Part print with two shaded views. Sizes in mm from the minimum x, y, z corner. Round coordinates to 2 decimals unless told otherwise and drop trailing zeros. Write each loop counter-clockwise with the first axis right and the second up, starting at its lowest first coordinate (ties: lowest second). Pieces come first, ordered by that corner, then holes. Notation, with made-up numbers: (42, 42) -> (52, 42) arc R18 cw to (52, 75) -> close; hole circle Ø3 at (70.25, -36.75). An arc over 180 degrees is marked (long way). Return JSON: item names as keys, results as strings. Group by question number.
(1) Saw through at A-A (x = 19.3). List the corners of the cut face in (y, z).
(2) Drill centre lines: L1, parallel to Y at x = 19.3, z = 2.6; L2, parallel to Y at x = 19.3, z = 0.7; L3, parallel to Y at x = 4, z = 2 (1 decimal). Where is each one in solid material? Low to high. Write a range as from..to.
(3) Mould opens along Y. For the marked faces 1, 2 and 3 say: +Y half, -Y half, draft (parallel to the pull), parting line (faces both ways), or undercut.
(4) Saw through at B-B (y = 19.3). List the corners of the cut face in (x, z).
(5) Saw through at C-C (z = 1.1). List the corners of the cut face in (x, y).
(6) Saw through at D-D (y = 28). List the corners of the cut face in (x, z) (1 decimal).
(7) Drop flat-ended pins along their axis: pin 1 Ø1 at (x, z) = (7, 0.5) entering from -Y; pin 2 Ø1 at (x, z) = (27.5, 2.5) entering from -Y; pin 3 Ø5 at (x, y) = (19.3, 19.3) entering from -Z. Give the stop position or say it passes through.
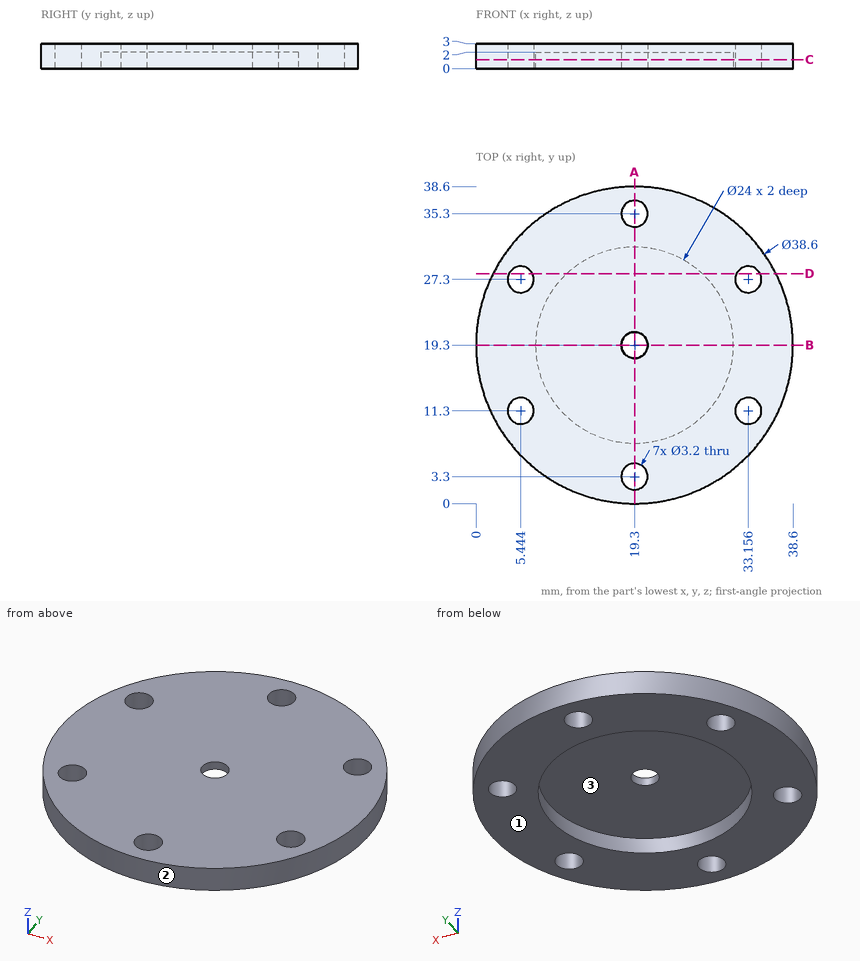
Computed values:
{
 "1": {"outline": "(0, 0) -> (1.7, 0) -> (1.7, 3) -> (0, 3) -> close; (4.9, 0) -> (7.3, 0) -> (7.3, 2) -> (17.7, 2) -> (17.7, 3) -> (4.9, 3) -> close; (20.9, 2) -> (31.3, 2) -> (31.3, 0) -> (33.7, 0) -> (33.7, 3) -> (20.9, 3) -> close; (36.9, 0) -> (38.6, 0) -> (38.6, 3) -> (36.9, 3) -> close"},
 "2": {"L1": "0..1.7, 4.9..17.7, 20.9..33.7, 36.9..38.6", "L2": "0..1.7, 4.9..7.3, 31.3..33.7, 36.9..38.6", "L3": "7.5..10.6, 12..26.6, 28..31.1"},
 "3": {"face 1": "draft", "face 2": "parting line", "face 3": "undercut"},
 "4": {"outline": "(0, 0) -> (7.3, 0) -> (7.3, 2) -> (17.7, 2) -> (17.7, 3) -> (0, 3) -> close; (20.9, 2) -> (31.3, 2) -> (31.3, 0) -> (38.6, 0) -> (38.6, 3) -> (20.9, 3) -> close"},
 "5": {"outline": "circle Ø38.6 at (19.3, 19.3); hole circle Ø3.2 at (5.44, 11.3); hole circle Ø3.2 at (5.44, 27.3); hole circle Ø24 at (19.3, 19.3); hole circle Ø3.2 at (19.3, 3.3); hole circle Ø3.2 at (19.3, 35.3); hole circle Ø3.2 at (33.16, 11.3); hole circle Ø3.2 at (33.16, 27.3)"},
 "6": {"outline": "(2.1, 0) -> (4, 0) -> (4, 3) -> (2.1, 3) -> close; (6.9, 0) -> (11, 0) -> (11, 2) -> (27.6, 2) -> (27.6, 0) -> (31.7, 0) -> (31.7, 3) -> (6.9, 3) -> close; (34.6, 0) -> (36.5, 0) -> (36.5, 3) -> (34.6, 3) -> close"},
 "7": {"pin 1": "y = 4.03", "pin 2": "y = 1.6", "pin 3": "z = 2"}
}
